Build history of the part. All positions in model axes, mm. A direction names the side the tool comes from. Coordinates: 2 decimals unless noted, no trailing zeros. Order: outer loops, then holes, each group sorted by start corner. A loop starts at its lowest first (then second) coordinate and runs counter-clockwise, first axis right, second up. Notation, with made-up numbers: M 18,-7 L 76,-7 A32 ccw 76,19 Z; hole C 7,-26 d4. An arc over 180 degrees is marked long. Use a Markdown table: item, result. Add a question column.
from build123d import *

# Parameters (mm, degrees)
F1_DEPTH = 21
F3_DEPTH = 42
F5_DEPTH = 50
F7_DEPTH = 50
F8_W     = 40
F8_H     = 8
F9_DEPTH = 40
F10_R    = 20
F11_SIZE = 5


with BuildPart() as f1:
    # F0 (on Right) → F1 (new body, symmetric)
    with BuildSketch(Plane.YZ):
        Polygon((40, 0), (0, 0), (-32, 0), (-40, 0), (-40, -1.9478090107), (40, -1.9478090107), align=None)
        Polygon((-32, 0), (0, 0), (40, 0), (40, 13), (30, 13), (30, 8), (-32, 8), align=None)
    extrude(amount=F1_DEPTH, both=True)

    # F2 (on face) → F3 (join)
    with BuildSketch(Plane(origin=(-21, 0, 0), x_dir=(0, -1, 0), z_dir=(-1, 0, 0))):
        Polygon((-30, 13), (-40, 13), (-40, -1.9478090107), (40, -1.9478090107), (40, 0), (32, 0), (10, 0), (10, 8), (-30, 8), align=None)
    extrude(amount=F3_DEPTH)

    # F4 (on face) → F5 (join)
    with BuildSketch(Plane(origin=(-63, 0, 0), x_dir=(0, -1, 0), z_dir=(-1, 0, 0))):
        Polygon((-40, 0), (-40, -1.9478090107), (40, -1.9478090107), (40, 0), (10, 0), align=None)
    extrude(amount=F5_DEPTH)

    # F6 (on face) → F7 (join)
    with BuildSketch(Plane(origin=(-63, 0, 0), x_dir=(0, -1, 0), z_dir=(-1, 0, 0))):
        Polygon((-30, 13), (-40, 13), (-40, 0), (-30, 0), (-30, 8), align=None)
    extrude(amount=F7_DEPTH)

    # F8 (on face) → F9 (join)
    with BuildSketch(Plane(origin=(-63, 0, 0), x_dir=(0, -1, 0), z_dir=(-1, 0, 0))):
        Polygon((-30, 13), (-30, 8), (10, 8), (10, 11.5), align=None)
        with Locations((-10, 4)):
            Rectangle(F8_W, F8_H)
    extrude(amount=F9_DEPTH)

    # F10
    f10_edges = [f1.edges().sort_by_distance(p)[0] for p in [
        (-103, -10, 5.75),
    ]]
    fillet(f10_edges, radius=F10_R)

    # F11
    f11_edges = [f1.edges().sort_by_distance(p)[0] for p in [
        (0, -32, 8),
    ]]
    chamfer(f11_edges, length=F11_SIZE)


solid = f1.part
(1) Drill centre lines: line 1 along Y through (x, z) = (-47, 7.5); line 2 along Z through (x, y) = (-17, -23.5); line 3 along Z through (x, y) = (-3, -35). Where is each one in solid material? Low to high. Write a range as from..to.
(2) Slice it at A-A on x = -23.5. Give the cut face in (y, z).
(3) Slice it at B-B on z = 9.75. Give the cut face in (x, y), and give its area (3 significant figures).
(4) Drop flat-ended pins along their axis: P1, Ø2, axis at y = 17, z = 9, coming from the -X side; P2, Ø12, axis at x = -89.5, y = -27.5, coming from the +Z side; P3, Ø2.5, axis at y = 18, z = 9.5, coming from the +X side. Give the stop position or say it passes through.
(5) Which spindle directions (+Z, -Z, +X, -X, +Y, -Y) get a long thin tool onto all of the face, cutting with end or side? Do faces 1 (the flat face through (0, -32, 2)), 2 (the flat face through (-45, 40, 6)), 3 (the flat face through (-20, 30, 10)), 4 (the flat face through (21, 8, 4)), 5 (the flat face through (-52, -10, 4)). Say none if no direction does.
(6) Slice it at D-D on x = -9. Give the cut face in (y, z), and give its area (3 significant figures).
(7) Slice it at C-C on y = -22. Give the cut face in (x, z).
Solutions:
| question | item | result |
|---|---|---|
| 1 | line 1 | -10..40 |
| 1 | line 2 | -1.95..8 |
| 1 | line 3 | -1.95..0 |
| 2 | outline | M -40,-1.95 L 40,-1.95 L 40,13 L 30,13 L 30,8 L -10,8 L -10,0 L -40,0 Z |
| 3 | outline | M -113,30 L -103,30 L -103,10 A20 ccw -83,-10 L -63,-10 L -63,30 L 21,30 L 21,40 L -113,40 Z |
| 3 | area | 2,850 mm² |
| 4 | P1 | x = -103 |
| 4 | P2 | z = 0 |
| 4 | P3 | x = -63 |
| 5 | face 1 | +Z, +X, -X, -Y |
| 5 | face 2 | +Z, -Z, +X, -X, +Y |
| 5 | face 3 | +Z, +X, -Y |
| 5 | face 4 | +Z, -Z, +X, +Y, -Y |
| 5 | face 5 | +Z, -X, -Y |
| 6 | outline | M -40,-1.95 L 40,-1.95 L 40,13 L 30,13 L 30,8 L -27,8 L -32,3 L -32,0 L -40,0 Z |
| 6 | area | 769 mm² |
| 7 | outline | M -113,-1.95 L 21,-1.95 L 21,8 L -21,8 L -21,0 L -113,0 Z |
